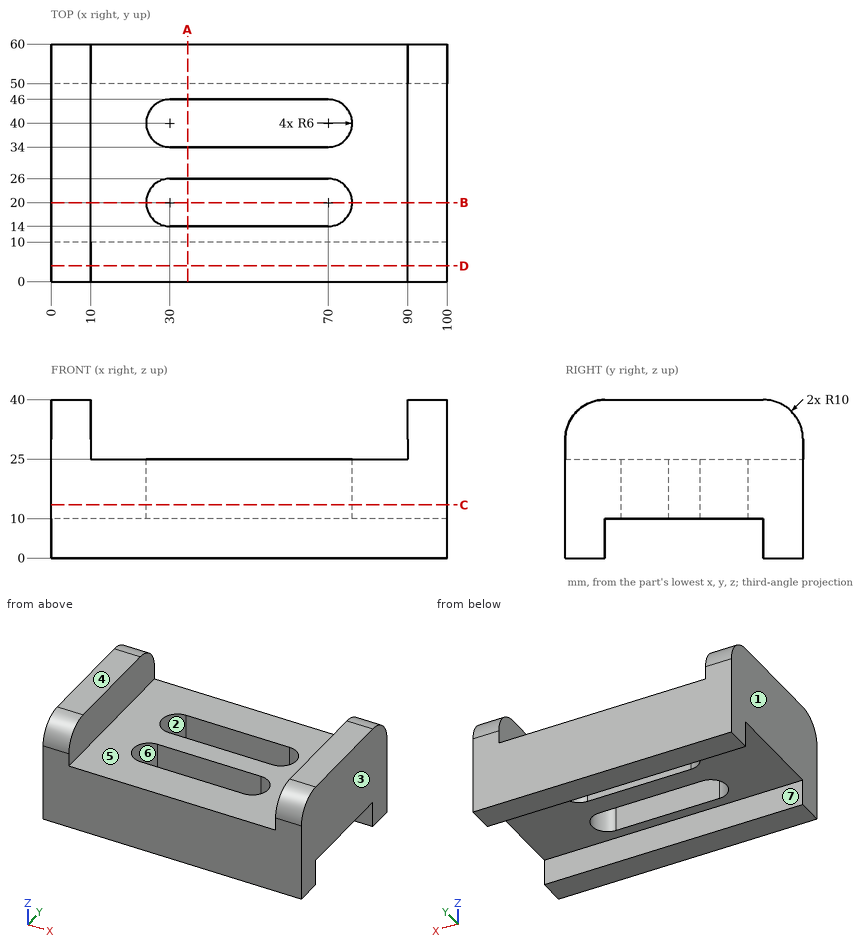
Input: dimensioned drawing with shaded views. Units: mm. Origin: part minimum x, y, z. A direction names the side the tool comes from. Coordinates: 2 decimals unless noted, no trailing zeros. Loops run counter-clockwise (first coordinate to the right, second up) from the corner with the lowest first, then second, coordinate; pieces in that order, holes last. Notation, with made-up numbers: (61.5, 12.5) -> (101.5, 12.5) arc R20 cw to (101.5, 32.5) -> close; hole circle Ø8 at (5, 87.5). An arc over 180 degrees is marked (long way). One line per item, written item: value. Start each with the question number.
Q1. Set-up query: the marked faces 5, 6 and 7. Return all of +Z, -Z, +X, -X, +Y, -Y with unobstructed straight access to the full face (end or side cutting, diameter ignored); none if empty.
Q2. Mould query, pull axis X, two halves, no side actions, for the marked faces 1, 2, 3 and 4. Classes: pulls with the +X half, pulls with the -X half, needs draft (parallel to the pull), parting line crosses it, or undercut.
Q3. Line query: line 1 along Y through (x, z) = (60.5, 24.5); line 2 along X through (y, z) = (36.5, 27); line 3 along Y through (x, z) = (89.5, 9.5). Output: solid intervals per line, ascending.
Q4. Contact query for flat-ended pins moving along their axis: P1, Ø2, axis at x = 55, z = 8.5, coming from the -Y side; P2, Ø12, axis at x = 52, y = 52.5, coming from the +Z side. Output: stop coordinate, or through.
Q5. Section query D-D, the plane y = 4. Return the cut outline in (x, z).
Q6. Section query B-B, the plane y = 20. Return the cut outline in (x, z), and give its area (3 significant figures).
Q7. Section query A-A, the plane x = 34.5. Return the cut outline in (y, z), and give its area (3 significant figures).
Q8. Section query C-C, the plane z = 13.5. Return the cut outline in (x, y).
Results:
1. face 5: +Z, +Y, -Y
1. face 6: +Z, -Z
1. face 7: -Z, +X, -X
2. face 1: pulls with the -X half
2. face 2: undercut
2. face 3: pulls with the +X half
2. face 4: needs draft
3. line 1: 0 to 14, 26 to 34, 46 to 60
3. line 2: 0 to 10, 90 to 100
3. line 3: 0 to 10, 50 to 60
4. P1: y = 0
4. P2: z = 25
5. outline: (0, 0) -> (100, 0) -> (100, 38) -> (90, 38) -> (90, 25) -> (10, 25) -> (10, 38) -> (0, 38) -> close
6. outline: (0, 10) -> (24, 10) -> (24, 25) -> (10, 25) -> (10, 40) -> (0, 40) -> close; (76, 10) -> (100, 10) -> (100, 40) -> (90, 40) -> (90, 25) -> (76, 25) -> close
6. area: 1,020 mm^2
7. outline: (0, 0) -> (10, 0) -> (10, 10) -> (14, 10) -> (14, 25) -> (0, 25) -> close; (26, 10) -> (34, 10) -> (34, 25) -> (26, 25) -> close; (46, 10) -> (50, 10) -> (50, 0) -> (60, 0) -> (60, 25) -> (46, 25) -> close
7. area: 740 mm^2
8. outline: (0, 0) -> (100, 0) -> (100, 60) -> (0, 60) -> close; hole (30, 14) -> (70, 14) arc R6 ccw to (70, 26) -> (30, 26) arc R6 ccw to start; hole (30, 34) -> (70, 34) arc R6 ccw to (70, 46) -> (30, 46) arc R6 ccw to start
